Design review of the part built by this model. Coordinates are the model's own, in mm. A direction names the side the tool comes from. Coordinates: 2 decimals unless noted, no trailing zeros. Order: outer loops, then holes, each group sorted by start corner. A loop starts at its lowest first (then second) coordinate and runs counter-clockwise, first axis right, second up. Notation, with made-up numbers: (68, 45.5) -> (116, 45.5) arc R24 cw to (116, 80.5) -> close; hole circle Ø6 at (53.25, -0.75). An arc over 180 degrees is marked (long way). Use a Markdown table: item, result. Add a question column.
Q1. Wall thickness on probe 1 along Y at (x, z) = (17.5, 2.5); probe 2 along X at (y, z) = (26, 6.5); probe 3 along X at (y, z) = (27, 9): over which ranges is each line inside the solid? List them lowest first.
Q2. The part is to be moulded in two halves that separate along X. For faces 3 (the face through (66, 17, 6)), 4 (the face through (61, 18, 8)), 5 (the face through (33, 18, 12)), say which applies: pulls with the +X half, pulls with the -X half, needs draft (parallel to the pull), parting line crosses it, or undercut.
Q3. Insertion check: pin 1 (2 mm diameter, centred on y = 12.5, z = 3.5, fed in from -X); pin 2 (1 mm diameter, centred on y = 29, z = 5, fed in from -X); pin 3 (2 mm diameter, centred on x = 41, y = 23.5, fed in from +Z). Each pin has a flat end and moves straight along its axis. Give the tip position at first contact, or say it passes through.
Q4. Machinability: for faces 1 (the face through (45.5, 18, 8)), 2 (the face through (40, 35, 6)), which of the approach directions +Z, -Z, +X, -X, +Y, -Y give a long, thin tool a straight path to every point of the face, cutting with its end or side? Answer none if there is none.
Q5. Add section D-D (x = 55). State the section outline as (y, z) points, then the cut area to 3 significant figures.
Q6. Add section C-C (z = 5). State the section outline as (x, y) points, then the cut area to 3 significant figures.
Q7. Add section A-A (y = 10). State the section outline as (x, z) points, then the cut area to 3 significant figures.
Q8. Add section B-B (x = 6). State the section outline as (y, z) points, then the cut area to 3 significant figures.
from build123d import *

# Parameters (mm, degrees)
F0_R     = 12.5
F1_DEPTH = 12
F2_W     = 10.5
F2_H     = 11


with BuildPart() as f1:
    # F0 (on Top) → F1 (new body)
    with BuildSketch(Plane.XY):
        with BuildLine():
            ThreePointArc((0, 17.5), (5.125631, 5.125631), (17.5, 0))
            Line((17.5, 0), (61, 0))
            ThreePointArc((61, 0), (64.535534, 1.464466), (66, 5))
            Line((66, 5), (66, 30))
            ThreePointArc((66, 30), (64.535534, 33.535534), (61, 35))
            Line((61, 35), (17.5, 35))
            ThreePointArc((17.5, 35), (5.125631, 29.874369), (0, 17.5))
        make_face()
        with Locations((17.5, 17.5)):
            Circle(F0_R, mode=Mode.SUBTRACT)
    extrude(amount=F1_DEPTH)

    # F2 (on face) → F3 (revolve, cut)
    with BuildSketch(Plane.XY.offset(12)):
        with Locations((40.25, 12)):
            Rectangle(F2_W, F2_H)
        with Locations((55.75, 12)):
            Rectangle(F2_W, F2_H)
    revolve(axis=Axis((40.25, 17.5, 12), (1, 0, 0)), mode=Mode.SUBTRACT)


solid = f1.part
Established:
| question | item | result |
|---|---|---|
| 1 | probe 1 | 0 to 5, 30 to 35 |
| 1 | probe 2 | 2.2 to 8.33, 26.67 to 35, 45.5 to 50.5, 61 to 66 |
| 1 | probe 3 | 2.8 to 9.38, 25.62 to 35, 45.5 to 50.5, 61 to 66 |
| 2 | face 3 | pulls with the +X half |
| 2 | face 4 | undercut |
| 2 | face 5 | needs draft |
| 3 | pin 1 | x = 0.46 |
| 3 | pin 2 | x = 3.89 |
| 3 | pin 3 | z = 3.51 |
| 4 | face 1 | +Z |
| 4 | face 2 | +Z, -Z, +X, -X, +Y |
| 5 | outline | (0, 0) -> (35, 0) -> (35, 12) -> (28.5, 12) arc R11 cw to (6.5, 12) -> (0, 12) -> close |
| 5 | area | 230 mm^2 |
| 6 | outline | (0, 17.5) arc R17.5 ccw to (17.5, 0) -> (61, 0) arc R5 ccw to (66, 5) -> (66, 30) arc R5 ccw to (61, 35) -> (17.5, 35) arc R17.5 ccw to start; hole circle Ø25 at (17.5, 17.5); hole (35, 9.01) -> (45.5, 9.01) -> (45.5, 25.99) -> (35, 25.99) -> close; hole (50.5, 9.01) -> (61, 9.01) -> (61, 25.99) -> (50.5, 25.99) -> close |
| 6 | area | 1,320 mm^2 |
| 7 | outline | (1.69, 0) -> (7.5, 0) -> (7.5, 12) -> (1.69, 12) -> close; (27.5, 0) -> (66, 0) -> (66, 12) -> (61, 12) -> (61, 3.95) -> (50.5, 3.95) -> (50.5, 12) -> (45.5, 12) -> (45.5, 3.95) -> (35, 3.95) -> (35, 12) -> (27.5, 12) -> close |
| 7 | area | 363 mm^2 |
| 8 | outline | (4.31, 0) -> (12.6, 0) -> (12.6, 12) -> (4.31, 12) -> close; (22.4, 0) -> (30.69, 0) -> (30.69, 12) -> (22.4, 12) -> close |
| 8 | area | 199 mm^2 |
